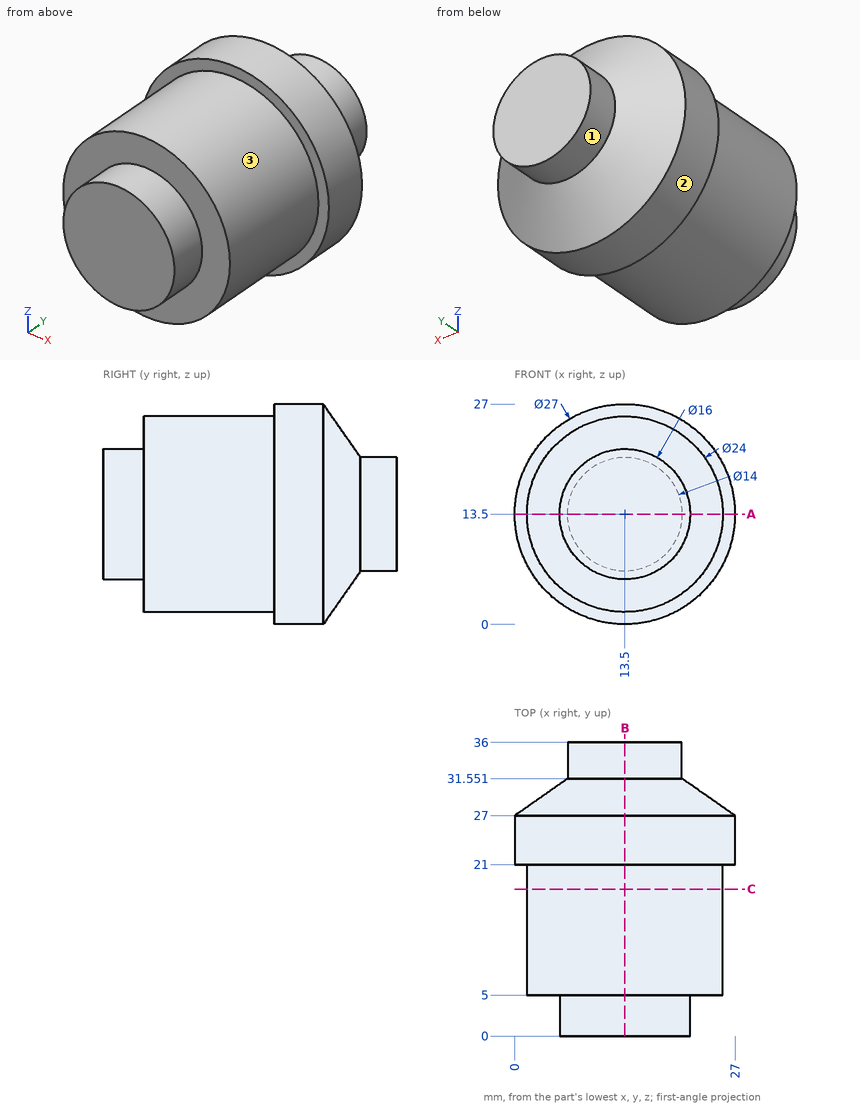
Design review of the part shown in the three views and the two pictorial views. Dimensions are in mm from the part's minimum x, y and z. A direction names the side the tool comes from. Coordinates: 2 decimals unless noted, no trailing zeros. Loops run counter-clockwise (first coordinate to the right, second up) from the corner with the lowest first, then second, coordinate; pieces in that order, holes last. Notation, with made-up numbers: M -37.75,71.25 L -31.75,71.25 A26 cw -31.75,86.25 Z; hole C 88,59 d8. An arc over 180 degrees is marked long. Put each result on its own line as item: value. Start each with the question number.
Q1. Clearance check with flat-ended pins moving along their axes: pin 1 (2 mm diameter, centred on x = 12, y = 29.5, fed in from +Z) (1 decimal); pin 2 (4 mm diameter, centred on x = 16, z = 16, fed in from -Y); pin 3 (2 mm diameter, centred on y = 18, z = 3, fed in from +X); pin 4 (1 mm diameter, centred on x = 16.5, y = 14, fed in from +Z). State where each tip first meets the part, or that it passes through.
Q2. Add section B-B (x = 13.5). Write out the cut boundary in (y, z).
Q3. For the marked faces 1, 2 and 3, list the 3-axis set-ups (+Z, -Z, +X, -X, +Y, -Y) from which the entire face can be reached by the end or side of a thin tool; tool diameter is ignored.
Q4. Wall thickness on line 1 (Z direction, x = 4, y = 12.5); line 2 (Y direction, x = 23.25, z = 17.5) (1 decimal); line 3 (Y direction, x = 2.5, z = 12.25): over which ranges is each line inside the solid? List them lowest first.
Q5. Add section A-A (z = 13.5). Write out the cut boundary in (x, y).
Q6. Add section C-C (y = 18). Write out the cut boundary in (x, z), and give its area (3 significant figures).
Answers:
1. pin 1: stops at z = 24.8
1. pin 2: stops at y = 0
1. pin 3: stops at x = 20.83
1. pin 4: stops at z = 25.24
2. outline: M 0,5.5 L 5,5.5 L 5,1.5 L 21,1.5 L 21,0 L 27,0 L 31.55,6.5 L 36,6.5 L 36,20.5 L 31.55,20.5 L 27,27 L 21,27 L 21,25.5 L 5,25.5 L 5,21.5 L 0,21.5 Z
3. face 1: +Y
3. face 2: +Y, -Y
3. face 3: -Y
4. line 1: z = 6.17 to 20.83
4. line 2: y = 5 to 29.1
4. line 3: y = 5 to 28.7
5. outline: M 0,21 L 1.5,21 L 1.5,5 L 5.5,5 L 5.5,0 L 21.5,0 L 21.5,5 L 25.5,5 L 25.5,21 L 27,21 L 27,27 L 20.5,31.55 L 20.5,36 L 6.5,36 L 6.5,31.55 L 0,27 Z
6. outline: C 13.5,13.5 d24
6. area: 452 mm^2
